The model under review builds one solid part; all positions refer to its coordinate system, in mm. A direction names the side the tool comes from. Give positions to 0.01 mm unless a question says otherwise; leave off trailing zeros. Order: outer loops, then holes, each group sorted by start corner. A loop starts at its lowest first (then second) coordinate and runs counter-clockwise, first axis right, second up. Notation, with made-up numbers: (59.5, 58) - (99.5, 58) arc R25 ccw to (99.5, 82) - close; hole circle Ø1 at (21.5, 32.25). An arc over 180 degrees is marked (long way). Use CSV: the item, a comma, the result in double quotes.
```python
from build123d import *

# Parameters (mm, degrees)
F0_R     = 3.81
F1_DEPTH = 25.4
F2_R     = 5.3793870979
F2_R_2   = 3.81
F3_DEPTH = 5.08
F4_R     = 3.81
F5_DEPTH = 2.54


with BuildPart() as f1:
    # F0 (on Top) → F1 (new body)
    with BuildSketch(Plane.XY):
        with Locations((10.3501314297, 0)):
            Circle(F0_R)
    extrude(amount=F1_DEPTH)

    # F2 (on face) → F3 (join)
    with BuildSketch(Plane.XY.offset(25.4)):
        with Locations((10.3501314297, 0)):
            Circle(F2_R)
        with Locations((10.3501314297, 0)):
            Circle(F2_R_2, mode=Mode.SUBTRACT)
        with Locations((10.3501314297, 0)):
            Circle(F2_R_2)
    extrude(amount=F3_DEPTH)

    # F4 (on face) → F5 (cut)
    with BuildSketch(Plane.XY.offset(30.48)):
        with Locations((10.3501314297, 0)):
            Circle(F4_R)
    extrude(amount=-F5_DEPTH, mode=Mode.SUBTRACT)


solid = f1.part
```
Item 1: Take a section at A-A, the plane y = 0. Give the boundary of the cut face in (x, z), and give its area (3 significant figures).
Results list:
outline,"(4.97, 25.4) - (6.54, 25.4) - (6.54, 0) - (14.16, 0) - (14.16, 25.4) - (15.73, 25.4) - (15.73, 30.48) - (14.16, 30.48) - (14.16, 27.94) - (6.54, 27.94) - (6.54, 30.48) - (4.97, 30.48) - close"
area,"229 mm2"
Item 2: Mouldability with a two-part tool opening along X and no side actions: class faces 1 (the face through (15.48, 1.62, 27.9)), 2 (the face through (10, 0, 27.94)), 3 (the face through (11, 4, 25.4)) as pulls with the +X half, pulls with the -X half, needs draft (parallel to the pull), parting line crosses it, or undercut.
Results list:
face 1,"parting line crosses it"
face 2,"undercut"
face 3,"needs draft"
Item 3: Wall thickness on L1, parallel to Z at x = 6, y = -3; L2, parallel to Y at x = 10.5, z = 5.5; L3, parallel to Z at x = 10.25, y = 3: over which ranges is each line inside the solid? List them lowest first.
Results list:
L1,"z = 25.4 to 30.48"
L2,"y = -3.81 to 3.81"
L3,"z = 0 to 27.94"
Item 4: Take a section at B-B, the plane x = 8.5. Give the boundary of the cut face in (y, z), and give its area (3 significant figures).
Results list:
outline,"(-5.05, 25.4) - (-3.33, 25.4) - (-3.33, 0) - (3.33, 0) - (3.33, 25.4) - (5.05, 25.4) - (5.05, 30.48) - (3.33, 30.48) - (3.33, 27.94) - (-3.33, 27.94) - (-3.33, 30.48) - (-5.05, 30.48) - close"
area,"204 mm2"
Item 5: Take a section at C-C, the plane z = 9.5. Give the boundary of the cut face in (x, y).
Results list:
outline,"circle Ø7.62 at (10.35, 0)"
Item 6: Clearance check with flat-ended pins moving along their axes: pin 1 (5 mm diameter, centred on x = 10.5, y = -2, fed in from -Z); pin 2 (2.5 mm diameter, centred on x = 10, y = -0.5, fed in from +Z); pin 3 (4 mm diameter, centred on y = 2, z = 22.5, fed in from -X). State where each tip first meets the part, or that it passes through.
Results list:
pin 1,"stops at z = 0"
pin 2,"stops at z = 27.94"
pin 3,"stops at x = 6.54"
Item 7: Tool access review of faces 4 (the face through (10, 0, 0)), 5 (the face through (13.984, 1.144, 12.522)), 6 (the face through (13.984, 1.144, 29.228)): name each direction out of +Z, -Z, +X, -X, +Y, -Y from which nothing blocks a thin tool from reaching the whole face with its end or side.
Results list:
face 4,"-Z, +X, -X, +Y, -Y"
face 5,"-Z"
face 6,"+Z"
Item 8: Take a section at D-D, the plane y = -4.5. Give the boundary of the cut face in (x, z).
Results list:
outline,"(7.4, 25.4) - (13.3, 25.4) - (13.3, 30.48) - (7.4, 30.48) - close"
